Check sheet for the modelled part. Datum: model origin and axes. Units: mm. A direction names the side the tool comes from. Round coordinates to 2 decimals unless told otherwise and drop trailing zeros. Order: outer loops, then holes, each group sorted by start corner. A loop starts at its lowest first (then second) coordinate and runs counter-clockwise, first axis right, second up. Notation, with made-up numbers: (49.5, 10.5) -> (92.5, 10.5) arc R13 ccw to (92.5, 26.5) -> close; hole circle Ø6 at (3.5, 54.5). An arc over 180 degrees is marked (long way). Answer in a Markdown table with one row per item. Add a question column.
1. Sectioned sample at B-B, the plane y = 33.5. Record the boundary of the cut face in (x, z), then the cut area to 3 significant figures.
2. Access from +Z, -Z, +X, -X, +Y, -Y to the whole of each face (thin tool, end or side, straight path). Record for faces 1 (the flat face through (37, 10, 4)), 2 (the flat face through (19, 22, 0)), 3 (the flat face through (7, 33, 4)).
3. Sectioned sample at C-C, the plane x = 7. Record the boundary of the cut face in (y, z), then the cut area to 3 significant figures.
4. Material ranges on L1, parallel to X at y = 35.5, z = 4; L2, parallel to Z at x = 37, y = 39; L3, parallel to Y at x = 37, z = 4, recorded low to high. Write a range as from..to.
5. Sectioned sample at A-A, the plane z = 4. Record the boundary of the cut face in (x, y).
6. Depth check by flat-ended pin: P1, Ø2, axis at x = 7, z = 3.5, coming from the +Y side; P2, Ø2, axis at x = 37, z = 3, coming from the -Y side. Enter the tip coordinate at first touch or a pass-through.
7. Draft check along Z on faces 4 (the cylindrical face through (41.1, 21.8, 7.14)), 5 (the flat face through (42, 21, 4)), 6 (the flat face through (7, 10, 4)). Enter one of: +Z half, -Z half, draft (parallel to the pull), parting line (faces both ways), or undercut.
```python
from build123d import *

# Parameters (mm, degrees)
SKETCH1_W           = 42
SKETCH1_H           = 43
BOSS_EXTRUDE1_DEPTH = 8
SKETCH2_R           = 2.1
CUT_EXTRUDE1_DEPTH  = 10
SKETCH3_R           = 2.1
CUT_EXTRUDE2_DEPTH  = 10
FILLET1_R           = 3


with BuildPart() as part:
    # Sketch1 → Boss-Extrude1 (new body)
    with BuildSketch(Plane.XY):
        with Locations((21, 21.5)):
            Rectangle(SKETCH1_W, SKETCH1_H)
    extrude(amount=BOSS_EXTRUDE1_DEPTH)

    # Sketch2 → Cut-Extrude1 (cut)
    with BuildSketch(Plane.XZ):
        with Locations((37, 4)):
            Circle(SKETCH2_R)
        with Locations((7, 4)):
            Circle(SKETCH2_R)
    extrude(amount=-CUT_EXTRUDE1_DEPTH, mode=Mode.SUBTRACT)

    # Sketch3 → Cut-Extrude2 (cut)
    with BuildSketch(Plane(origin=(0, 43, 0), x_dir=(1, 0, 0), z_dir=(0, 1, 0))):
        with Locations((37, -4)):
            Circle(SKETCH3_R)
        with Locations((7, -4)):
            Circle(SKETCH3_R)
    extrude(amount=-CUT_EXTRUDE2_DEPTH, mode=Mode.SUBTRACT)

    # Fillet1
    fillet1_edges = [part.edges().sort_by_distance(p)[0] for p in [
        (42, 21.5, 8),
        (42, 21.5, 0),
    ]]
    fillet(fillet1_edges, radius=FILLET1_R)


solid = part.part
```
Answer key:
| question | item | result |
|---|---|---|
| 1 | outline | (0, 0) -> (39, 0) arc R3 ccw to (42, 3) -> (42, 5) arc R3 ccw to (39, 8) -> (0, 8) -> close; hole circle Ø4.2 at (7, 4); hole circle Ø4.2 at (37, 4) |
| 1 | area | 304 mm² |
| 2 | face 1 | -Y |
| 2 | face 2 | -Z, +X, -X, +Y, -Y |
| 2 | face 3 | +Y |
| 3 | outline | (0, 0) -> (43, 0) -> (43, 1.9) -> (33, 1.9) -> (33, 6.1) -> (43, 6.1) -> (43, 8) -> (0, 8) -> (0, 6.1) -> (10, 6.1) -> (10, 1.9) -> (0, 1.9) -> close |
| 3 | area | 260 mm² |
| 4 | L1 | x = 0..4.9, 9.1..34.9, 39.1..42 |
| 4 | L2 | z = 0..1.9, 6.1..8 |
| 4 | L3 | y = 10..33 |
| 5 | outline | (0, 0) -> (4.9, 0) -> (4.9, 10) -> (9.1, 10) -> (9.1, 0) -> (34.9, 0) -> (34.9, 10) -> (39.1, 10) -> (39.1, 0) -> (42, 0) -> (42, 43) -> (39.1, 43) -> (39.1, 33) -> (34.9, 33) -> (34.9, 43) -> (9.1, 43) -> (9.1, 33) -> (4.9, 33) -> (4.9, 43) -> (0, 43) -> close |
| 6 | P1 | stops at y = 33 |
| 6 | P2 | stops at y = 10 |
| 7 | face 4 | +Z half |
| 7 | face 5 | draft |
| 7 | face 6 | undercut |
